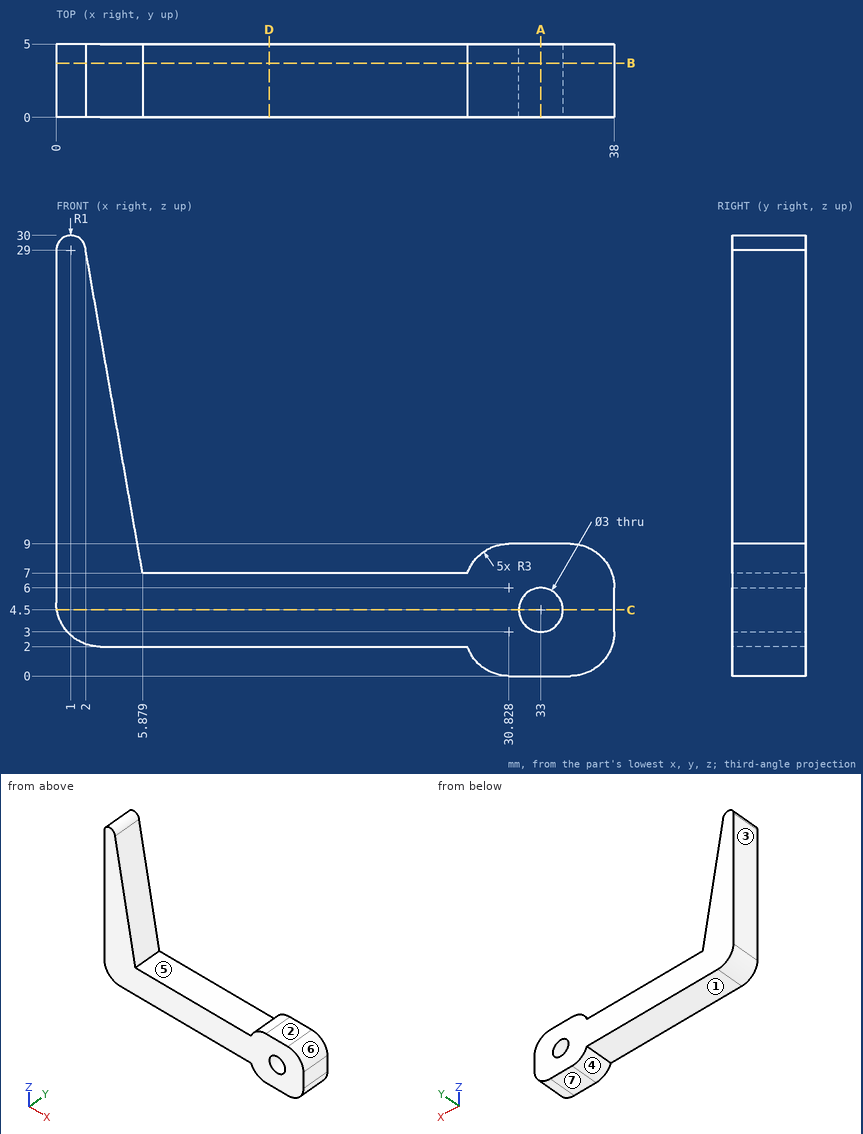
Here's the drawing with two shaded views (mm, measured from the low corner). I have some questions. A direction names the side the tool comes from. Coordinates: 2 decimals unless noted, no trailing zeros. Write each loop counter-clockwise with the first axis right and the second up, starting at its lowest first coordinate (ties: lowest second). Pieces come first, ordered by that corner, then holes. Notation, with made-up numbers: (-20.75, -31) -> (-1.75, -31) arc R18 ccw to (-1.75, -24) -> close; hole circle Ø4 at (-6, 16). An arc over 180 degrees is marked (long way). Use a Markdown table: item, result. Add a question column.
(1) Please list where these lines run through material, in increasing order: line 1 (Z direction, x = 33, y = 1.45); line 2 (Z direction, x = 21.5, y = 4.6); line 3 (Z direction, x = 35, y = 3.65).
(2) For the marked faces 1, 2 and 3, which set-ups out of +Z, -Z, +X, -X, +Y, -Y let a thin tool reach every point of the face, with its end or its side?
(3) If we section it at D-D, the plane x = 14.5: Write out the boundary of the cut face in (y, z), and give its area (3 significant figures).
(4) If we section it at C-C, the plane z = 4.5: Write out the boundary of the cut face in (x, y).
(5) I'm going to push flat-ended pins straight in: P1, Ø1.5, axis at x = 14, y = 3, coming from the -Z side; P2, Ø2.5, axis at x = 16, y = 2, coming from the +Z side. Where does each tip first touch, or does it pass through?
(6) We'd pull the mould along X, two halves only. Please class the marked faces 4, 5, 6 and 7: +X half, -X half, draft (parallel to the pull), parting line (faces both ways), or undercut.
(7) If we section it at A-A, the plane x = 33: Write out the boundary of the cut face in (y, z).
(8) If we section it at B-B, the plane y = 3.7: Write out the boundary of the cut face in (x, z).
Outcome:
| question | item | result |
|---|---|---|
| 1 | line 1 | z = 0 to 3, 6 to 9 |
| 1 | line 2 | z = 2 to 7 |
| 1 | line 3 | z = 0 to 9 |
| 2 | face 1 | -Z, -X, +Y, -Y |
| 2 | face 2 | +Z, +X, +Y, -Y |
| 2 | face 3 | +Z, -Z, -X, +Y, -Y |
| 3 | outline | (0, 2) -> (5, 2) -> (5, 7) -> (0, 7) -> close |
| 3 | area | 25.0 mm^2 |
| 4 | outline | (0.04, 0) -> (31.5, 0) -> (31.5, 5) -> (0.04, 5) -> close; (34.5, 0) -> (38, 0) -> (38, 5) -> (34.5, 5) -> close |
| 5 | P1 | stops at z = 2 |
| 5 | P2 | stops at z = 7 |
| 6 | face 4 | -X half |
| 6 | face 5 | undercut |
| 6 | face 6 | +X half |
| 6 | face 7 | draft |
| 7 | outline | (0, 0) -> (5, 0) -> (5, 3) -> (0, 3) -> close; (0, 6) -> (5, 6) -> (5, 9) -> (0, 9) -> close |
| 8 | outline | (0, 5) arc R3 ccw to (3, 2) -> (28, 2) arc R3 ccw to (30.83, 0) -> (35, 0) arc R3 ccw to (38, 3) -> (38, 6) arc R3 ccw to (35, 9) -> (30.83, 9) arc R3 ccw to (28, 7) -> (5.88, 7) -> (2, 29) arc R1 ccw to (0, 29) -> close; hole circle Ø3 at (33, 4.5) |
